```python
from build123d import *

# Parameters (mm, degrees)
F0_W     = 1000
F0_H     = 500
F1_DEPTH = 25
F2_W     = 100
F2_H     = 100
F3_DEPTH = 700
F5_D     = 50
F7_D     = 50
F9_D     = 50


with BuildPart() as f1:
    # F0 (on Top) → F1 (new body)
    with BuildSketch(Plane.XY):
        with Locations((3.7799999118, 20.495297656)):
            Rectangle(F0_W, F0_H)
    extrude(amount=F1_DEPTH)

    # F2 (on face) → F3 (join)
    with BuildSketch(Plane(origin=(0, 0, 0), x_dir=(1, 0, 0), z_dir=(0, 0, -1))):
        with Locations((-396.2200000882, 129.504702344)):
            Rectangle(F2_W, F2_H)
    extrude(amount=F3_DEPTH)

    # F5 (through all)
    with Locations(Plane.XZ.offset(179.504702344)):
        with Locations((-396.2200000882, -500)):
            Hole(F5_D / 2)

    # F7 (through all)
    with Locations(Plane.XZ.offset(179.504702344)):
        with Locations((-396.2200000882, -300)):
            Hole(F7_D / 2)

    # F9 (through all)
    with Locations(Plane.XZ.offset(179.504702344)):
        with Locations((-396.2200000882, -100)):
            Hole(F9_D / 2)

    # F12: F1 across plane


with BuildPart() as f1_1:
    add(f1.part)
    add(f1.part.mirror(Plane(origin=(3.7799999118, 270.495297656, 12.5), x_dir=(-1, 0, 0), z_dir=(0, 1, 0))))

    # F14: F1 across plane


with BuildPart() as f1_2:
    add(f1_1.part)
    add(f1_1.part.mirror(Plane(origin=(503.7799999118, 270.495297656, 12.5), x_dir=(0, 1, 0), z_dir=(1, 0, 0))))


solid = f1_2.part
```
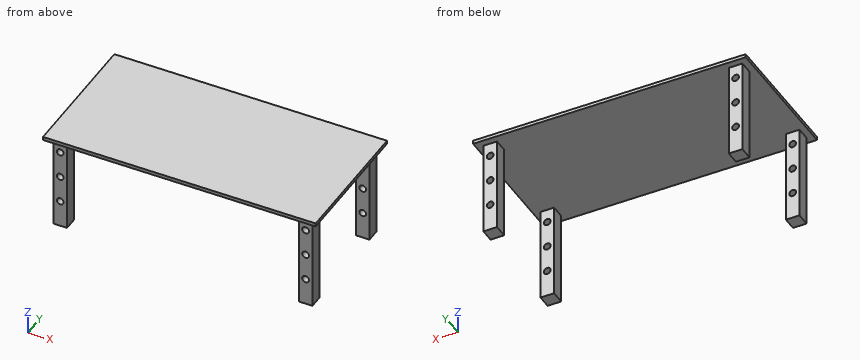
The model under review builds one solid part; all positions refer to its coordinate system, in mm. Coordinates: 2 decimals unless noted, no trailing zeros. Order: outer loops, then holes, each group sorted by start corner. A loop starts at its lowest first (then second) coordinate and runs counter-clockwise, first axis right, second up. Notation, with made-up numbers: (-0.5, 47) -> (27.5, 47) arc R30 ccw to (27.5, 70) -> close; hole circle Ø10 at (-30.75, -16). An arc over 180 degrees is marked (long way). Answer in a Markdown table with one row per item. Add a question column.
Item 1: Clearance check with flat-ended pins moving along their axes: pin 1 (4 mm diameter, centred on y = 661.5, z = -208, fed in from +X); pin 2 (1 mm diameter, centred on x = 1009, y = 406.5, fed in from -Z). State where each tip first meets the part, or that it passes through.
Item 2: We need section B-B on z = -417. Write out the cut boundary in (x, y), plus the area to 3 significant figures.
Item 3: We need section C-C on y = -143. Write out the cut boundary in (x, z), plus the area to 3 significant figures.
Item 4: We need section A-A on z = -100. Give the number of separate pieces and of enclosed holes in the cut face, plus the area to 3 significant figures.
Item 5: To check wall thickness, follow probe 1 along Z at (x, y) = (-396, 687); probe 2 along X at (y, z) = (-154.5, -99); probe 3 along X at (y, z) = (-146, -569). State the ranges of each line that lie inside material, in increasing order.
Final values:
| question | item | result |
|---|---|---|
| 1 | pin 1 | stops at x = 1453.78 |
| 1 | pin 2 | stops at z = 0 |
| 2 | outline | (-446.22, -179.5) -> (-346.22, -179.5) -> (-346.22, -79.5) -> (-446.22, -79.5) -> close; (-446.22, 620.5) -> (-346.22, 620.5) -> (-346.22, 720.5) -> (-446.22, 720.5) -> close; (1353.78, -179.5) -> (1453.78, -179.5) -> (1453.78, -79.5) -> (1353.78, -79.5) -> close; (1353.78, 620.5) -> (1453.78, 620.5) -> (1453.78, 720.5) -> (1353.78, 720.5) -> close |
| 2 | area | 40,000 mm2 |
| 3 | outline | (-496.22, 0) -> (-446.22, 0) -> (-446.22, -700) -> (-346.22, -700) -> (-346.22, 0) -> (1353.78, 0) -> (1353.78, -700) -> (1453.78, -700) -> (1453.78, 0) -> (1503.78, 0) -> (1503.78, 25) -> (-496.22, 25) -> close; hole circle Ø50 at (-396.22, -500); hole circle Ø50 at (-396.22, -300); hole circle Ø50 at (-396.22, -100); hole circle Ø50 at (1403.78, -500); hole circle Ø50 at (1403.78, -300); hole circle Ø50 at (1403.78, -100) |
| 3 | area | 178,000 mm2 |
| 4 | separate pieces | 8 |
| 4 | enclosed holes | 0 |
| 4 | area | 20,000 mm2 |
| 5 | probe 1 | z = -700 to -525, -475 to -325, -275 to -125, -75 to 25 |
| 5 | probe 2 | x = -446.22 to -421.2, -371.24 to -346.22, 1353.78 to 1378.8, 1428.76 to 1453.78 |
| 5 | probe 3 | x = -446.22 to -346.22, 1353.78 to 1453.78 |
